Can you work these out from the model? Positions are in its coordinate system, mm. A direction names the side the tool comes from. Give positions to 0.01 mm unless a question says otherwise; leave off trailing zeros. Order: outer loops, then holes, each group sorted by start corner. A loop starts at its lowest first (then second) coordinate and runs counter-clockwise, first axis right, second up. Notation, with made-up numbers: (-6, 53.5) - (52, 53.5) arc R23 cw to (52, 70.5) - close; hole circle Ø5 at (24, 82.25). An arc over 180 degrees is marked (long way). One line per question, with ' | ' between items.
```python
from build123d import *

# Parameters (mm, degrees)
BOSS_EXTRUDE1_DEPTH = 3
CUT_EXTRUDE1_REACH  = 58.648
SKETCH2_W           = 45
SKETCH2_H           = 26
CUT_EXTRUDE2_REACH  = 58.648
SKETCH4_R           = 2
CUT_EXTRUDE3_DEPTH  = 10


with BuildPart() as part:
    # Sketch1 → Boss-Extrude1 (new body)
    with BuildSketch(Plane.XY):
        with BuildLine():
            Line((10, 29.342801502), (10, 38.729833462))
            ThreePointArc((10, 38.729833462), (0, 40), (-10, 38.729833462))
            Line((-10, 38.729833462), (-10, 29.342801502))
            ThreePointArc((-10, 29.342801502), (-21.920310217, 21.920310217), (-29.342801502, 10))
            Line((-29.342801502, 10), (-38.729833462, 10))
            ThreePointArc((-38.729833462, 10), (-40, 0), (-38.729833462, -10))
            Line((-38.729833462, -10), (-29.342801502, -10))
            ThreePointArc((-29.342801502, -10), (-21.920310217, -21.920310217), (-10, -29.342801502))
            Line((-10, -29.342801502), (-10, -38.729833462))
            ThreePointArc((-10, -38.729833462), (0, -40), (10, -38.729833462))
            Line((10, -38.729833462), (10, -29.342801502))
            ThreePointArc((10, -29.342801502), (21.920310217, -21.920310217), (29.342801502, -10))
            Line((29.342801502, -10), (38.729833462, -10))
            ThreePointArc((38.729833462, -10), (40, 0), (38.729833462, 10))
            Line((38.729833462, 10), (29.342801502, 10))
            ThreePointArc((29.342801502, 10), (21.920310217, 21.920310217), (10, 29.342801502))
        make_face()
    extrude(amount=BOSS_EXTRUDE1_DEPTH)

    # Sketch2 → Cut-Extrude1 (cut, up to next)
    with BuildSketch(Plane.XY.offset(3), mode=Mode.PRIVATE) as cut_extrude1_sk1:
        Rectangle(SKETCH2_W, SKETCH2_H)
    cut_extrude1_tool1 = extrude(cut_extrude1_sk1.sketch, amount=-CUT_EXTRUDE1_REACH, mode=Mode.PRIVATE) & part.part
    add(cut_extrude1_tool1.solids().sort_by_distance((0, 0, 3))[0], mode=Mode.SUBTRACT)

    # Sketch3 → Cut-Extrude2 (cut, up to next)
    with BuildSketch(Plane.XY.offset(3), mode=Mode.PRIVATE) as cut_extrude2_sk1:
        with BuildLine():
            Line((-10.5, 21), (-10.5, 13))
            Line((-10.5, 13), (-14.5, 13))
            Line((-14.5, 13), (-14.5, 21))
            ThreePointArc((-14.5, 21), (-12.5, 23), (-10.5, 21))
        make_face()
    cut_extrude2_tool1 = extrude(cut_extrude2_sk1.sketch, amount=-CUT_EXTRUDE2_REACH, mode=Mode.PRIVATE) & part.part
    # Sketch3 → Cut-Extrude2 (cut, up to next)
    with BuildSketch(Plane.XY.offset(3), mode=Mode.PRIVATE) as cut_extrude2_sk2:
        with BuildLine():
            Line((10.5, 21), (10.5, 13))
            Line((10.5, 13), (14.5, 13))
            Line((14.5, 13), (14.5, 21))
            ThreePointArc((14.5, 21), (12.5, 23), (10.5, 21))
        make_face()
    cut_extrude2_tool2 = extrude(cut_extrude2_sk2.sketch, amount=-CUT_EXTRUDE2_REACH, mode=Mode.PRIVATE) & part.part
    add(cut_extrude2_tool1.solids().sort_by_distance((-12.5, 17.795808, 3))[0], mode=Mode.SUBTRACT)
    add(cut_extrude2_tool2.solids().sort_by_distance((12.5, 17.795808, 3))[0], mode=Mode.SUBTRACT)

    # Sketch4 → Cut-Extrude3 (cut)
    with BuildSketch(Plane.XY.offset(3)):
        with Locations((0, 35)):
            Circle(SKETCH4_R)
        with Locations((35, 0)):
            Circle(SKETCH4_R)
        with Locations((0, -35)):
            Circle(SKETCH4_R)
        with Locations((-35, 0)):
            Circle(SKETCH4_R)
    extrude(amount=-CUT_EXTRUDE3_DEPTH, mode=Mode.SUBTRACT)


solid = part.part
```
(1) On a 3-axis mill with a long thin cutter (end or side, diameter ignored), from which of +Z, -Z, +X, -X, +Y, -Y can I reach the whole of each face in a straight line? I mean faces 4 (the face through (-34, 10, 1)), 5 (the face through (-10, -34, 1)), 6 (the face through (-19, 13, 2)). Say none if no direction works.
Answer below:
face 4: +Z, -Z, -X, +Y | face 5: +Z, -Z, -X, -Y | face 6: +Z, -Z
(2) If we mould it in two halves opening along Y, with no side actions, what happens to faces 1 (the face through (21.78, -22.06, 1.48)), 2 (the face through (0, 40, 1)), 3 (the face through (-12.5, 23, 1.5))? For each: released by +Y, released by -Y, zero draft, split by the parting line, or undercut.
Answer below:
face 1: released by -Y | face 2: released by +Y | face 3: undercut
(3) If I drill on line 1 (Y direction, x = 0, z = 0.65); line 2 (Y direction, x = 35, z = 1.5); line 3 (Y direction, x = -1.5, z = 0.3), over which ranges is the centre line in solid material (lowest first)?
Answer below:
line 1: -40 to -37, -33 to -13, 13 to 33, 37 to 40 | line 2: -10 to -2, 2 to 10 | line 3: -39.97 to -36.32, -33.68 to -13, 13 to 33.68, 36.32 to 39.97
(4) Imagine slicing it at C-C (y = 0). List the corners of the cut face in (x, z) for me.
Answer below:
outline: (-40, 0) - (-37, 0) - (-37, 3) - (-40, 3) - close; (-33, 0) - (-22.5, 0) - (-22.5, 3) - (-33, 3) - close; (22.5, 0) - (33, 0) - (33, 3) - (22.5, 3) - close; (37, 0) - (40, 0) - (40, 3) - (37, 3) - close
(5) Will these pins go through, and if not, where does the flat tip stop? pin 1 (0.9 mm diameter, centred on y = 33, z = 2, fed in from +X); pin 2 (0.9 mm diameter, centred on x = -18.5, z = 2, fed in from -Y); pin 3 (1 mm diameter, centred on x = 19, z = 2, fed in from +Y).
Answer below:
pin 1: x = 10 | pin 2: y = -25.2 | pin 3: y = 24.87
(6) Imagine slicing it at B-B (z = 1.1). Count the separate pieces of the cut face and the enclosed holes in it, and give its area (3 significant figures).
Answer below:
separate pieces: 1 | enclosed holes: 5 | area: 2,450 mm^2
(7) Imagine slicing it at D-D (x = 0). List the corners of the cut face in (y, z) for me, and give its area (3 significant figures).
Answer below:
outline: (-40, 0) - (-37, 0) - (-37, 3) - (-40, 3) - close; (-33, 0) - (-13, 0) - (-13, 3) - (-33, 3) - close; (13, 0) - (33, 0) - (33, 3) - (13, 3) - close; (37, 0) - (40, 0) - (40, 3) - (37, 3) - close | area: 138 mm^2
(8) Imagine slicing it at A-A (x = -35). List the corners of the cut face in (y, z) for me.
Answer below:
outline: (-10, 0) - (-2, 0) - (-2, 3) - (-10, 3) - close; (2, 0) - (10, 0) - (10, 3) - (2, 3) - close
